Here's how the part is built. I have some questions about the finished solid (model axes, mm). Face numbers are marked on the shaded views. A direction names the side the tool comes from. Round coordinates to 2 decimals unless told otherwise and drop trailing zeros. Order: outer loops, then holes, each group sorted by start corner. A loop starts at its lowest first (then second) coordinate and runs counter-clockwise, first axis right, second up.
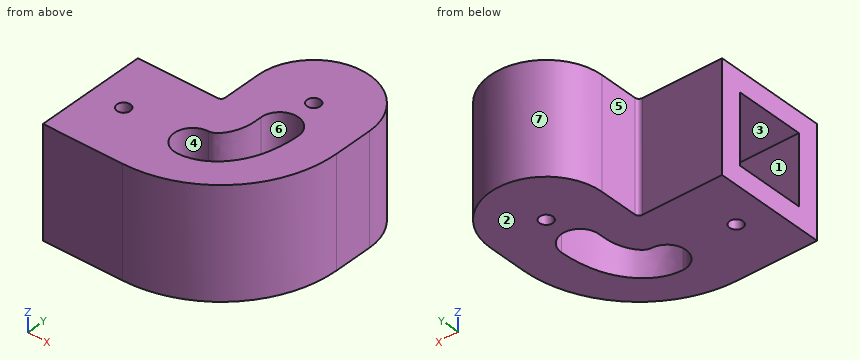
```python
from build123d import *

# Parameters (mm, degrees)
SKETCH1_R           = 2.5
BOSS_EXTRUDE1_DEPTH = 41.4
SKETCH2_W           = 26
SKETCH2_H           = 26
CUT_EXTRUDE1_DEPTH  = 31
CUT_EXTRUDE4_DEPTH  = 41.4
SKETCH4_R           = 2.5
BOSS_EXTRUDE2_DEPTH = 0.4


with BuildPart() as part:
    # Sketch1 → Boss-Extrude1 (new body)
    with BuildSketch(Plane.XY):
        with BuildLine():
            Line((8.125515238, 31.748109782), (-21.874484762, 31.748109782))
            Line((-21.874484762, 31.748109782), (-21.874484762, -10.251890218))
            Line((-21.874484762, -10.251890218), (8.125515238, -10.251890218))
            ThreePointArc((8.125515238, -10.251890218), (38.88466022, 2.488964801), (51.625515238, 33.248109782))
            Line((51.625515238, 33.248109782), (51.625515238, 47.748109782))
            ThreePointArc((51.625515238, 47.748109782), (30.625515238, 68.748109782), (9.625515238, 47.748109782))
            Line((9.625515238, 47.748109782), (9.625515238, 33.248109782))
            ThreePointArc((9.625515238, 33.248109782), (9.18617541, 32.18744961), (8.125515238, 31.748109782))
        make_face()
        with Locations((-9.374484762, 10.748109782)):
            Circle(SKETCH1_R, mode=Mode.SUBTRACT)
        with Locations((30.625515238, 47.748109782)):
            Circle(SKETCH1_R, mode=Mode.SUBTRACT)
    extrude(amount=BOSS_EXTRUDE1_DEPTH)

    # Sketch2 → Cut-Extrude1 (cut)
    with BuildSketch(Plane.ZY.offset(21.874484762)):
        with Locations((20.7, 10.748109782)):
            Rectangle(SKETCH2_W, SKETCH2_H)
    extrude(amount=-CUT_EXTRUDE1_DEPTH, mode=Mode.SUBTRACT)

    # Sketch3 → Cut-Extrude4 (cut)
    with BuildSketch(Plane.XY.offset(41.4)):
        with BuildLine():
            ThreePointArc((23.625515238, 32.748109782), (30.625515238, 39.748109782), (37.625515238, 32.748109782))
            add(Edge.make_bspline(
                [(16.625515238, 3.748109782), (24.940509595, 3.748109782), (36.171087452, 14.120308293), (37.625515238, 29.35283955), (37.625515238, 32.748109782)],
                knots=[0, 0, 0, 0, 0.619735212, 1, 1, 1, 1], degree=3))
            ThreePointArc((16.625515238, 3.748109782), (9.625515238, 10.748109782), (16.625515238, 17.748109782))
            add(Edge.make_bspline(
                [(16.625515238, 17.748109782), (19.461751307, 17.748109782), (23.882566791, 24.826419712), (23.625515238, 30.398814735), (23.625515238, 32.748109782)],
                knots=[0, 0, 0, 0, 0.571663187, 1, 1, 1, 1], degree=3))
        make_face()
    extrude(amount=-CUT_EXTRUDE4_DEPTH, mode=Mode.SUBTRACT)

    # Sketch4 → Boss-Extrude2 (add)
    with BuildSketch(Plane(origin=(0, 0, 33.7), x_dir=(-1, 0, 0), z_dir=(0, 0, -1))):
        with Locations((9.374484762, 10.748109782)):
            Circle(SKETCH4_R)
    extrude(amount=-BOSS_EXTRUDE2_DEPTH)


solid = part.part
```
1. If we section it at D-D, the plane x = -8: Write out the boundary of the cut face in (y, z), and give its area (3 significant figures).
Evaluation:
outline: (-10.25, 0) - (8.66, 0) - (8.66, 7.7) - (-2.25, 7.7) - (-2.25, 33.7) - (23.75, 33.7) - (23.75, 7.7) - (12.84, 7.7) - (12.84, 0) - (31.75, 0) - (31.75, 41.4) - (12.84, 41.4) - (12.84, 34.1) - (8.66, 34.1) - (8.66, 41.4) - (-10.25, 41.4) - close
area: 1,000 mm2
2. If we mould it in two halves opening along Z, with no side actions, what happens to the marked faces 1, 2, 3 and 4? For each: released by +Z, released by -Z, zero draft, split by the parting line, or undercut.
Evaluation:
face 1: undercut
face 2: released by -Z
face 3: undercut
face 4: zero draft
3. I need wall thicknesses on probe 1 along Y at (x, z) = (7, 12); probe 2 along X at (y, z) = (11.5, 38.5); probe 3 along X at (y, z) = (45, 29). Which ranges of each line are inside material? Lowest first, please.
Evaluation:
probe 1: y = -10.25 to -2.25, 23.75 to 31.75
probe 2: x = -21.87 to -11.76, -6.99 to 9.67, 31.17 to 45.8
probe 3: x = 9.63 to 51.63
4. If we section it at C-C, the plane z = 15: State how many separate pieces and enclosed holes the cut face has, and give its area (3 significant figures).
Evaluation:
separate pieces: 1
enclosed holes: 2
area: 2,670 mm2
5. If we section it at A-A, the plane x = -17: Write out the boundary of the cut face in (y, z).
Evaluation:
outline: (-10.25, 0) - (31.75, 0) - (31.75, 41.4) - (-10.25, 41.4) - close; hole (-2.25, 7.7) - (23.75, 7.7) - (23.75, 33.7) - (-2.25, 33.7) - close
6. I'm going to push flat-ended pins straight in: P1, Ø3, axis at x = -9.37, y = 10.75, coming from the -Z side; P2, Ø10, axis at y = 59.5, z = 17, coming from the -X side; P3, Ø5, axis at y = 50.5, z = 21.5, coming from the -X side; P4, Ø12, axis at x = 1, y = 53.5, coming from the -Z side. Where does each tip first touch, or does it pass through?
Evaluation:
P1: stops at z = 33.7
P2: stops at x = 10.74
P3: stops at x = 9.63
P4: passes through
7. On a 3-axis mill with a long thin cutter (end or side, diameter ignored), from which of +Z, -Z, +X, -X, +Y, -Y can I reach the whole of each face in a straight line? I mean the marked faces 5, 6 and 7. Say none if no direction works.
Evaluation:
face 5: +Z, -Z, -X, +Y
face 6: +Z, -Z
face 7: +Z, -Z, +Y
8. If we section it at B-B, the plane x = 14.5: Write out the boundary of the cut face in (y, z), and give its area (3 significant figures).
Evaluation:
outline: (-9.78, 0) - (4.08, 0) - (4.08, 41.4) - (-9.78, 41.4) - close; (17.42, 0) - (61.2, 0) - (61.2, 41.4) - (17.42, 41.4) - close
area: 2,390 mm2
